Input: part model. Units: mm. Frame: model coordinates. A direction names the side the tool comes from. Give positions to 0.01 mm unless a question says otherwise; leave off trailing zeros. Order: outer loops, then holes, each group sorted by start corner. A loop starts at its lowest first (then second) coordinate and runs counter-clockwise, first axis right, second up. Notation, with made-up numbers: (-6.75, 25) - (17.25, 25) arc R32 cw to (17.25, 58) - close; hole circle Ø3 at (34.5, 29.25). An arc over 180 degrees is marked (long way). Answer in a Markdown table with one row per item. Add a question column.
1. Section query A-A on x = -16.5. Return loops of the section in (y, z), and give its area (3 significant figures).
2. Contact query for flat-ended pins moving along their axis: pin 1 (1 mm diameter, centred on y = -2.5, z = -5, fed in from -X); pin 2 (4.5 mm diameter, centred on y = 2, z = -1.5, fed in from -X). Output: stop coordinate, or through.
3. Mould query, pull axis Y, two halves, no side actions, for faces 1 (the face through (-11, 6.5, 0)), 2 (the face through (-11.5, -5.5, -4.5)), 3 (the face through (7.232, 0, 0)). Classes: released by +Y, released by -Y, zero draft, split by the parting line, or undercut.
4. Section query B-B on y = -5. Return loops of the section in (x, z).
5. Section query C-C on z = 0.5. Return loops of the section in (x, y), and give its area (3 significant figures).
6. Section query D-D on z = -1. Return loops of the section in (x, y).
7. Ray query, line 1 (Y direction, x = -9, z = -1); line 2 (Z direction, x = 6, y = 3); line 3 (Z direction, x = -5.5, y = 0). Return the intervals inside material, ascending. Write a range as [from, to].
8. Access query for faces 4 (the face through (-11, 0, 6.5)), 5 (the face through (-11, -4.5, -5.5)), 6 (the face through (4.232, 0, 1)). Directions: +Z, -Z, +X, -X, +Y, -Y. A direction counts if a zero-diameter tool reaches every point of the face in a straight line with its end or side. Return the directions, or none.
```python
from build123d import *

# Parameters (mm, degrees)
F0_W     = 32
F0_H     = 9
F0_W_2   = 1
F1_DEPTH = 6.5
F2_DEPTH = 5.5
F3_DEPTH = 7
F4_W     = 1
F4_H     = 1
F5_DEPTH = 35
F8_DEPTH = 2
F4_W_2   = 9
F9_DEPTH = 35


with BuildPart() as f1:
    # F0 (on Top) → F1 (new body)
    with BuildSketch(Plane.XY):
        Polygon((4.2322745472, -4.5), (-27.7677254528, -4.5), (-28.7677254528, -4.5), (-28.7677254528, -6.5), (7.2322745472, -6.5), (7.2322745472, 6.5), (-28.7677254528, 6.5), (-28.7677254528, 4.5), (-27.7677254528, 4.5), (4.2322745472, 4.5), align=None)
        with Locations((-11.7677254528, 0)):
            Rectangle(F0_W, F0_H)
        with Locations((-28.2677254528, 0)):
            Rectangle(F0_W_2, F0_H)
    extrude(amount=F1_DEPTH)

    # F0 (on Top) → F2 (cut)
    with BuildSketch(Plane.XY):
        with Locations((-11.7677254528, 0)):
            Rectangle(F0_W, F0_H)
    extrude(amount=F2_DEPTH, mode=Mode.SUBTRACT)

    # F0 (on Top) → F3 (join)
    with BuildSketch(Plane.XY):
        Polygon((4.2322745472, -4.5), (-27.7677254528, -4.5), (-28.7677254528, -4.5), (-28.7677254528, -6.5), (7.2322745472, -6.5), (7.2322745472, 6.5), (-28.7677254528, 6.5), (-28.7677254528, 4.5), (-27.7677254528, 4.5), (4.2322745472, 4.5), align=None)
    extrude(amount=-F3_DEPTH)

    # F4 (on face) → F5 (cut)
    with BuildSketch(Plane(origin=(-28.7677254528, 0, 0), x_dir=(0, -1, 0), z_dir=(-1, 0, 0))):
        with Locations((-5, -4.5)):
            Rectangle(F4_W, F4_H)
    extrude(amount=-F5_DEPTH, mode=Mode.SUBTRACT)

    # F6: F1 across plane


with BuildPart() as f1_1:
    add(f1.part)
    add(f1.part.mirror(Plane.XZ), mode=Mode.INTERSECT)

    # F7 (on face) → F8 (cut)
    with BuildSketch(Plane(origin=(4.2322745472, 0, 0), x_dir=(0, -1, 0), z_dir=(-1, 0, 0))):
        Polygon((4.5, -4), (-4.5, -4), (-4.5, -5), (-4.5, -7), (4.5, -7), (4.5, -5), align=None)
    extrude(amount=-F8_DEPTH, mode=Mode.SUBTRACT)

    # F4 (on face) → F9 (join, through all)
    with BuildSketch(Plane(origin=(-28.7677254528, 0, 0), x_dir=(0, -1, 0), z_dir=(-1, 0, 0))):
        with Locations((0, -6.5)):
            Rectangle(F4_W_2, F4_H)
    extrude(amount=-F9_DEPTH)


solid = f1_1.part
```
Answer:
| question | item | result |
|---|---|---|
| 1 | outline | (-6.5, -7) - (6.5, -7) - (6.5, 6.5) - (-6.5, 6.5) - close; hole (-5.5, -5) - (-4.5, -5) - (-4.5, -6) - (4.5, -6) - (4.5, -5) - (5.5, -5) - (5.5, -4) - (4.5, -4) - (4.5, 5.5) - (-4.5, 5.5) - (-4.5, -4) - (-5.5, -4) - close |
| 1 | area | 70.0 mm² |
| 2 | pin 1 | stops at x = 6.23 |
| 2 | pin 2 | stops at x = -28.77 |
| 3 | face 1 | released by +Y |
| 3 | face 2 | undercut |
| 3 | face 3 | zero draft |
| 4 | outline | (-28.77, -7) - (7.23, -7) - (7.23, 6.5) - (-28.77, 6.5) - (-28.77, -4) - (6.23, -4) - (6.23, -5) - (-28.77, -5) - close |
| 5 | outline | (-28.77, -6.5) - (7.23, -6.5) - (7.23, 6.5) - (-28.77, 6.5) - close; hole (-27.77, -4.5) - (4.23, -4.5) - (4.23, 4.5) - (-27.77, 4.5) - close |
| 5 | area | 180 mm² |
| 6 | outline | (-28.77, -6.5) - (7.23, -6.5) - (7.23, 6.5) - (-28.77, 6.5) - (-28.77, 4.5) - (4.23, 4.5) - (4.23, -4.5) - (-28.77, -4.5) - close |
| 7 | line 1 | y = [-6.5, -4.5], [4.5, 6.5] |
| 7 | line 2 | z = [-7, -6], [-4, 6.5] |
| 7 | line 3 | z = [-7, -6], [5.5, 6.5] |
| 8 | face 4 | +Z, +X, -X, +Y, -Y |
| 8 | face 5 | -X |
| 8 | face 6 | none |
